Part model, mm, in its own coordinate system. A direction names the side the tool comes from. Give positions to 0.01 mm unless a question says otherwise; leave off trailing zeros. Order: outer loops, then holes, each group sorted by start corner. A loop starts at its lowest first (then second) coordinate and runs counter-clockwise, first axis right, second up. Notation, with made-up numbers: M -16.5,9 L 7.5,9 A18 cw 7.5,42 Z; hole C 24.5,63 d8. An arc over 180 degrees is marked long. Return JSON: item names as keys, results as strings.
from build123d import *

# Parameters (mm, degrees)
F0_W     = 27
F0_H     = 25
F1_DEPTH = 40
F2_R     = 5
F3_R     = 7.5
F4_DEPTH = 10
F5_W     = 40
F5_H     = 40
F6_DEPTH = 10
F7_SIZE  = 1
F8_R     = 5
F9_DEPTH = 10


with BuildPart() as f1:
    # F0 (on Top) → F1 (new body)
    with BuildSketch(Plane.XY):
        with Locations((0, 12.5)):
            Rectangle(F0_W, F0_H)
    extrude(amount=F1_DEPTH)

    # F2
    f2_edges = [f1.edges().sort_by_distance(p)[0] for p in [
        (13.5, 25, 20),
        (-13.5, 25, 20),
    ]]
    fillet(f2_edges, radius=F2_R)

    # F3 (on face) → F4 (join)
    with BuildSketch(Plane(origin=(0, 25, 0), x_dir=(-1, 0, 0), z_dir=(0, 1, 0))):
        with Locations((0, 20)):
            Circle(F3_R)
    extrude(amount=F4_DEPTH)

    # F5 (on face) → F6 (join)
    with BuildSketch(Plane(origin=(0, 35, 0), x_dir=(-1, 0, 0), z_dir=(0, 1, 0))):
        with Locations((0, 20)):
            Rectangle(F5_W, F5_H)
    extrude(amount=F6_DEPTH)

    # F7
    f7_edges = [f1.edges().sort_by_distance(p)[0] for p in [
        (-20, 45, 20),
        (0, 45, 40),
        (20, 45, 20),
        (0, 45, 0),
        (-20, 35, 20),
        (0, 35, 40),
        (0, 35, 0),
        (20, 35, 20),
    ]]
    chamfer(f7_edges, length=F7_SIZE)

    # F8 (on face) → F9 (cut)
    with BuildSketch(Plane(origin=(0, 45, 0), x_dir=(-1, 0, 0), z_dir=(0, 1, 0))):
        with Locations((-9, 29)):
            Circle(F8_R)
        with Locations((9, 29)):
            Circle(F8_R)
        with Locations((-9, 11)):
            Circle(F8_R)
        with Locations((9, 11)):
            Circle(F8_R)
    extrude(amount=-F9_DEPTH, mode=Mode.SUBTRACT)


solid = f1.part
Q1. Band-saw the part on B-B (z = 11). Give the cut face in (x, y).
Established:
{"outline": "M -20,36 L -19,35 L -14,35 L -14,45 L -19,45 L -20,44 Z; M -13.5,0 L 13.5,0 L 13.5,20 A5 ccw 8.5,25 L -8.5,25 A5 ccw -13.5,20 Z; M -4,35 L 4,35 L 4,45 L -4,45 Z; M 14,35 L 19,35 L 20,36 L 20,44 L 19,45 L 14,45 Z"}
Q2. Probe line 1 along Z through (x, y) = (-9, 38); line 2 along X through (y, z) = (38, 26.5); line 3 along Y through (x, z) = (-8, 6). List the from-to ranges inside material, lowest first.
Established:
{"line 1": "z = 0 to 6, 16 to 24, 34 to 40", "line 2": "x = -20 to -13.33, -4.67 to 4.67, 13.33 to 20", "line 3": "y = 0 to 25, 35 to 45"}
Q3. Two-plate mould, pull along X, no slides. Class faces 5 (the flat face through (-13.5, 10, 20)), 6 (the cylindrical face through (-13.77, 40.07, 12.5)), 7 (the flat face through (-8, 25, 20)): +X half, -X half, draft (parallel to the pull), parting line (faces both ways), or undercut.
Established:
{"face 5": "-X half", "face 6": "undercut", "face 7": "draft"}
Q4. Band-saw the part on D-D (z = 20). Give the cut face in (x, y), then the cut area to 3 significant figures.
Established:
{"outline": "M -20,36 L -19,35 L -7.5,35 L -7.5,25 L -8.5,25 A5 ccw -13.5,20 L -13.5,0 L 13.5,0 L 13.5,20 A5 ccw 8.5,25 L 7.5,25 L 7.5,35 L 19,35 L 20,36 L 20,44 L 19,45 L -19,45 L -20,44 Z", "area": "1,210 mm²"}
Q5. Band-saw the part on C-C (x = 5). Give the cut face in (y, z).
Established:
{"outline": "M 0,0 L 25,0 L 25,14.41 L 35,14.41 L 35,14 L 45,14 L 45,26 L 35,26 L 35,25.59 L 25,25.59 L 25,40 L 0,40 Z; M 35,1 L 36,0 L 44,0 L 45,1 L 45,8 L 35,8 Z; M 35,32 L 45,32 L 45,39 L 44,40 L 36,40 L 35,39 Z"}
Q6. Band-saw the part on A-A (y = 42.5). Give the cut face in (x, z).
Established:
{"outline": "M -20,0 L 20,0 L 20,40 L -20,40 Z; hole C -9,11 d10; hole C -9,29 d10; hole C 9,11 d10; hole C 9,29 d10"}
Q7. Pin check, flat tips, straight feed: pin 1 (1 mm diameter, centred on y = 19, z = 34, fed in from +X); pin 2 (22 mm diameter, centred on y = 13, z = 10.5, fed in from -X). Stop position of each tip, or through.
Established:
{"pin 1": "stops at x = 13.5", "pin 2": "stops at x = -13.5"}
Q8. 3-axis set-ups, long thin cutter, end or side, ignore diameter. For faces 1 (the cylindrical face through (-12.07, 23.5, 20.28)), 2 (the flat face through (9, 35, 20)), 3 (the flat face through (13.5, 10, 20)), 4 (the cylindrical face through (4.23, 40.07, 12.5)): which of +Z, -Z, +X, -X, +Y, -Y reach the whole face in a straight line?
Established:
{"face 1": "+Z, -Z, -X", "face 2": "none", "face 3": "+Z, -Z, +X, -Y", "face 4": "+Y"}
